The listing builds one solid part. Answer for the finished solid, in the listing's coordinates (mm). A direction names the side the tool comes from. Coordinates: 2 decimals unless noted, no trailing zeros. Order: outer loops, then holes, each group sorted by start corner. A loop starts at its lowest first (then second) coordinate and runs counter-clockwise, first axis right, second up. Notation, with made-up numbers: (70.25, -23) -> (94.25, -23) arc R21 ccw to (94.25, 3) -> close; hole circle Ø2 at (42.25, 38). An arc over 180 degrees is marked (long way). Answer in a Markdown table with one row per item.
```python
from build123d import *

# Parameters (mm, degrees)
PAD_DEPTH           = 20
POCKET_DEPTH        = 18.5
POCKET001_DEPTH     = 5
LINEARPATTERN_COUNT = 10
LINEARPATTERN_PITCH = 4.444444
PAD001_DEPTH        = 15.5
SKETCH004_R         = 1.69
POCKET002_DEPTH     = 6
SKETCH005_W         = 20
SKETCH005_H         = 4.8
POCKET003_DEPTH     = 0.6
SKETCH006_R         = 0.5
SKETCH006_W         = 10.6
SKETCH006_H         = 6
POCKET004_DEPTH     = 5


with BuildPart() as part:
    # Sketch → Pad (new body)
    with BuildSketch(Plane.XY):
        with BuildLine():
            Line((-17, 32), (17, 32))
            ThreePointArc((22, 27), (20.535534, 30.535534), (17, 32))
            Line((22, 27), (22, -27))
            ThreePointArc((17, -32), (20.535534, -30.535534), (22, -27))
            Line((17, -32), (-17, -32))
            ThreePointArc((-22, -27), (-20.535534, -30.535534), (-17, -32))
            Line((-22, -27), (-22, 27))
            ThreePointArc((-17, 32), (-20.535534, 30.535534), (-22, 27))
        make_face()
    extrude(amount=PAD_DEPTH)

    # Sketch001 (on Face10 of Pad) → Pocket (cut)
    with BuildSketch(Plane.XY.offset(20)):
        with BuildLine():
            Line((-17, 30), (17, 30))
            ThreePointArc((20, 27), (19.12132, 29.12132), (17, 30))
            Line((20, 27), (20, -27))
            ThreePointArc((17, -30), (19.12132, -29.12132), (20, -27))
            Line((17, -30), (-17, -30))
            ThreePointArc((-20, -27), (-19.12132, -29.12132), (-17, -30))
            Line((-20, -27), (-20, 27))
            ThreePointArc((-17, 30), (-19.12132, 29.12132), (-20, 27))
        make_face()
    extrude(amount=-POCKET_DEPTH, mode=Mode.SUBTRACT)

    # Sketch002 (on Face4 of Pocket) → Pocket001 (cut)
    with BuildSketch(Plane(origin=(0, 0, 0), x_dir=(1, 0, 0), z_dir=(0, 0, -1))):
        with BuildLine():
            ThreePointArc((-15, 21), (-16, 20), (-15, 19))
            Line((-15, 19), (15, 19))
            ThreePointArc((15, 19), (16, 20), (15, 21))
            Line((15, 21), (-15, 21))
        make_face()
    pocket001 = extrude(amount=-POCKET001_DEPTH, mode=Mode.SUBTRACT)

    # LinearPattern: Pocket001 ×10
    with Locations(*[(0, i * LINEARPATTERN_PITCH, 0) for i in range(1, LINEARPATTERN_COUNT)]):
        add(pocket001, mode=Mode.SUBTRACT)

    # Sketch003 (on Face59 of LinearPattern) → Pad001 (join)
    with BuildSketch(Plane.XY.offset(1.5)):
        with BuildLine():
            Line((-17, 30), (-13, 30))
            Line((-13, 30), (-13, 26))
            ThreePointArc((-16, 23), (-13.87868, 23.87868), (-13, 26))
            Line((-16, 23), (-20, 23))
            Line((-20, 27), (-20, 23))
            ThreePointArc((-17, 30), (-19.12132, 29.12132), (-20, 27))
        make_face()
        with BuildLine():
            Line((13, 30), (17, 30))
            ThreePointArc((20, 27), (19.12132, 29.12132), (17, 30))
            Line((20, 27), (20, 23))
            Line((20, 23), (16, 23))
            ThreePointArc((13, 26), (13.87868, 23.87868), (16, 23))
            Line((13, 26), (13, 30))
        make_face()
        with BuildLine():
            Line((-21, -23), (-17, -23))
            ThreePointArc((-13, -27), (-14.171573, -24.171573), (-17, -23))
            Line((-13, -27), (-13, -31))
            Line((-13, -31), (-17, -31))
            ThreePointArc((-21, -27), (-19.828427, -29.828427), (-17, -31))
            Line((-21, -27), (-21, -23))
        make_face()
        with BuildLine():
            Line((16, -23), (20, -23))
            Line((20, -23), (20, -27))
            ThreePointArc((16, -31), (18.828427, -29.828427), (20, -27))
            Line((16, -31), (12, -31))
            Line((12, -31), (12, -27))
            ThreePointArc((16, -23), (13.171573, -24.171573), (12, -27))
        make_face()
    extrude(amount=PAD001_DEPTH)

    # Sketch004 (on Face69 of Pad001) → Pocket002 (cut)
    with BuildSketch(Plane.XY.offset(17)):
        with Locations((16.5, 26.5)):
            Circle(SKETCH004_R)
        with Locations((-16.5, 26.5)):
            Circle(SKETCH004_R)
        with Locations((-16.5, -26.5)):
            Circle(SKETCH004_R)
        with Locations((16.5, -26.5)):
            Circle(SKETCH004_R)
    extrude(amount=-POCKET002_DEPTH, mode=Mode.SUBTRACT)

    # Sketch005 (on Face6 of Pocket002) → Pocket003 (cut)
    with BuildSketch(Plane.XZ.offset(32)):
        with Locations((0, 14.4)):
            Rectangle(SKETCH005_W, SKETCH005_H)
    extrude(amount=-POCKET003_DEPTH, mode=Mode.SUBTRACT)

    # Sketch006 (on Face6 of Pocket003) → Pocket004 (cut)
    with BuildSketch(Plane.XZ.offset(32)):
        with Locations((7.65, 14.4)):
            Circle(SKETCH006_R)
        with Locations((-7.65, 14.4)):
            Circle(SKETCH006_R)
        with Locations((0, 14.4)):
            Rectangle(SKETCH006_W, SKETCH006_H)
    extrude(amount=-POCKET004_DEPTH, mode=Mode.SUBTRACT)


solid = part.part
```
(1) A cutting plane is placed at D-D, the plane x = -3.5. Count the separate pieces of the cut face and the enclosed holes in it, then the cut area to 3 significant figures.
Check values:
| item | result |
|---|---|
| separate pieces | 12 |
| enclosed holes | 0 |
| area | 128 mm² |
(2) Which of the six approach directions +Z, -Z, +X, -X, +Y, -Y give full straight-line access (tool end or side, diameter ignored) to faces 4 (the flat face through (-20, 0, 11)), 5 (the cylindrical face through (-16, 6.64, 0.74))?
Check values:
| item | result |
|---|---|
| face 4 | +Z |
| face 5 | +Z, -Z |
(3) A cutting plane is placed at C-C, the plane y = 18. Determine the outline of the cut face in (x, z), then the cut area to 3 significant figures.
Check values:
| item | result |
|---|---|
| outline | (-22, 0) -> (22, 0) -> (22, 20) -> (20, 20) -> (20, 1.5) -> (-20, 1.5) -> (-20, 20) -> (-22, 20) -> close |
| area | 140 mm² |
(4) A cutting plane is placed at A-A, the plane z = 5. Determine the outline of the cut face in (x, y), then the cut area to 3 significant figures.
Check values:
| item | result |
|---|---|
| outline | (-22, -27) arc R5 ccw to (-17, -32) -> (17, -32) arc R5 ccw to (22, -27) -> (22, 27) arc R5 ccw to (17, 32) -> (-17, 32) arc R5 ccw to (-22, 27) -> close; hole (-20, -23) -> (-17, -23) arc R4 cw to (-13, -27) -> (-13, -30) -> (12, -30) -> (12, -27) arc R4 cw to (16, -23) -> (20, -23) -> (20, 23) -> (16, 23) arc R3 cw to (13, 26) -> (13, 30) -> (-13, 30) -> (-13, 26) arc R3 cw to (-16, 23) -> (-20, 23) -> close |
| area | 587 mm² |
(5) For a pull along Y with two mould halves and no side action, classify faces 1 (the flat face through (-22, 0, 10)), 2 (the cylindrical face through (-16, -20, 1)), 3 (the cylindrical face through (-21, -30, 10)) as released by +Y, released by -Y, zero draft, split by the parting line, or undercut.
Check values:
| item | result |
|---|---|
| face 1 | zero draft |
| face 2 | undercut |
| face 3 | released by -Y |
(6) Find the intervals of material crossed by line 1 along Y through (x, z) = (16.5, 15.4); line 2 along Y through (x, z) = (14, 17.75); line 3 along Z through (x, y) = (7.65, -30.65), in increasing order. Write a range as from..to.
Check values:
| item | result |
|---|---|
| line 1 | -32..-28.19, -24.81..-23, 23..24.81, 28.19..32 |
| line 2 | -32..-30, 30..32 |
| line 3 | 0..13.9, 14.9..20 |
(7) Flat-ended cylindrical pins translate along their axes: pin 1 (5.5 mm diameter, centred on x = 15.5, y = 27, fed in from +Z); pin 2 (5 mm diameter, centred on x = 12.5, y = -18, fed in from +Z); pin 3 (2 mm diameter, centred on y = -31.5, z = 13.5, fed in from -X). Find the tip coordinate at first contact, or state that the pin passes through.
Check values:
| item | result |
|---|---|
| pin 1 | z = 17 |
| pin 2 | z = 1.5 |
| pin 3 | x = -20.57 |
(8) A cutting plane is placed at B-B, the plane y = -20. Determine the outline of the cut face in (x, z).
Check values:
| item | result |
|---|---|
| outline | (-22, 0) -> (-16, 0) -> (-16, 1.5) -> (-20, 1.5) -> (-20, 20) -> (-22, 20) -> close; (16, 0) -> (22, 0) -> (22, 20) -> (20, 20) -> (20, 1.5) -> (16, 1.5) -> close |
